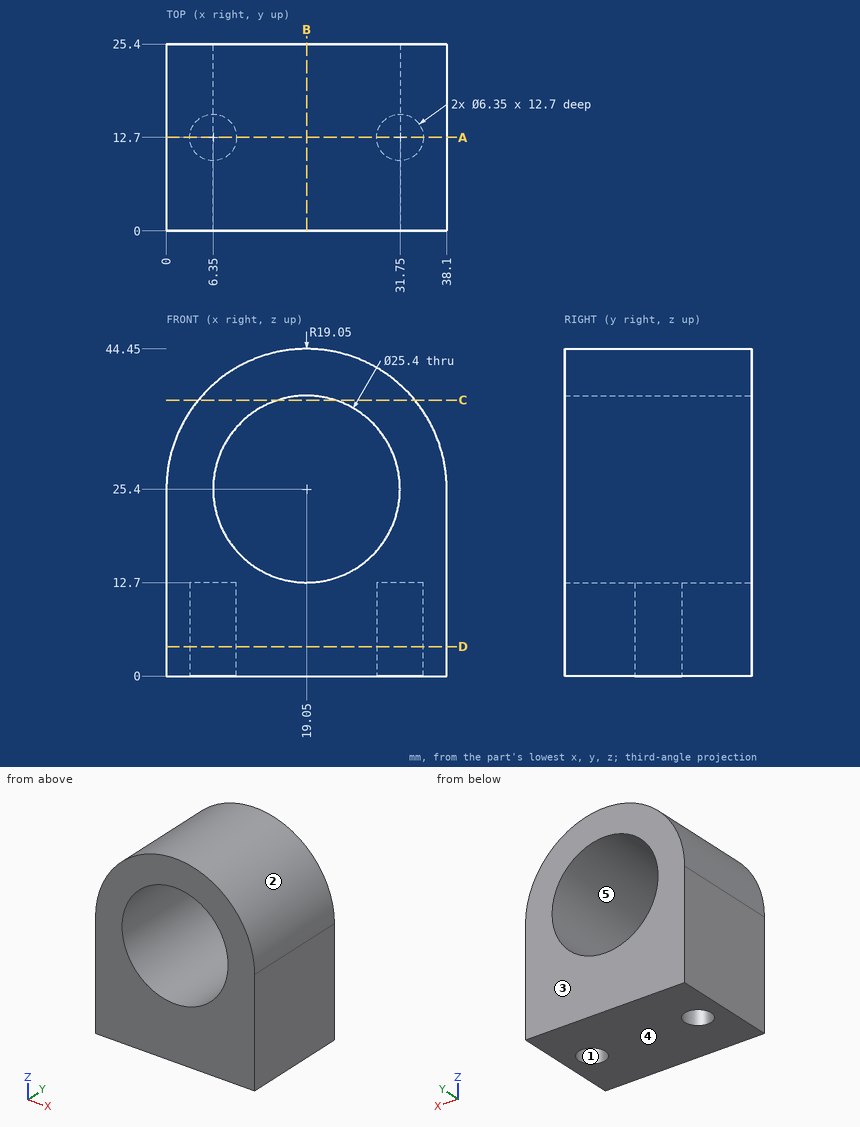
Geometry check sheet. Reference: drawing and pictorial views, mm from the part's lowest x, y, z. A direction names the side the tool comes from. Round coordinates to 2 decimals unless told otherwise and drop trailing zeros. Order: outer loops, then holes, each group sorted by start corner. A loop starts at its lowest first (then second) coordinate and runs counter-clockwise, first axis right, second up. Notation, with made-up numbers: M 22,-13.5 L 53,-13.5 A29 ccw 53,23.5 Z; hole C 42,49 d8. An arc over 180 degrees is marked long. One line per item, written item: value. Start each with the question number.
1. Gauge pin test, flat ends, axial feed: P1, Ø10, axis at x = 8, z = 20, coming from the -Y side; P2, Ø6, axis at x = 33.5, y = 11, coming from the +Z side (3 decimals); P3, Ø1, axis at x = 23, y = 18, coming from the +Z side (3 decimals); P4, Ø12, axis at x = 18, y = 14, coming from the +Z side. Record the tip position at first contact, or that the pin passes through.
2. Section check B-B on x = 19.05. Enter the section's corners in (y, z), and give its area (3 significant figures).
3. Section check C-C on z = 37.5. Enter the section's corners in (x, y), and give its area (3 significant figures).
4. Scan lines: line 1 along X through (y, z) = (12.7, 6.25) (3 decimals); line 2 along Y through (x, z) = (31.75, 7.5) (3 decimals); line 3 along Z through (x, y) = (19.05, 8.5). Record each from-to range of solid material in increasing order.
5. Section check A-A on y = 12.7. Enter the section's corners in (x, z) (3 decimals).
6. Section check D-D on z = 4. Enter the section's corners in (x, y) (3 decimals).
7. Access from +Z, -Z, +X, -X, +Y, -Y to the whole of each face (thin tool, end or side, straight path). Record for the marked faces 1 and 2.
8. Release check for a two-part mould opening along Z. For the marked faces 3, 4 and 5 record: released by +Z, released by -Z, zero draft, split by the parting line, or undercut.
Results found:
1. P1: y = 0
1. P2: z = 40.625
1. P3: z = 44.135
1. P4: z = 44.45
2. outline: M 0,0 L 25.4,0 L 25.4,12.7 L 0,12.7 Z; M 0,38.1 L 25.4,38.1 L 25.4,44.45 L 0,44.45 Z
2. area: 484 mm^2
3. outline: M 4.34,0 L 15.19,0 L 15.19,25.4 L 4.34,25.4 Z; M 22.91,0 L 33.76,0 L 33.76,25.4 L 22.91,25.4 Z
3. area: 551 mm^2
4. line 1: 0 to 3.175, 9.525 to 28.575, 34.925 to 38.1
4. line 2: 0 to 9.525, 15.875 to 25.4
4. line 3: 0 to 12.7, 38.1 to 44.45
5. outline: M 0,0 L 3.175,0 L 3.175,12.7 L 9.525,12.7 L 9.525,0 L 28.575,0 L 28.575,12.7 L 34.925,12.7 L 34.925,0 L 38.1,0 L 38.1,25.4 A19.05 ccw 0,25.4 Z; hole C 19.05,25.4 d25.4
6. outline: M 0,0 L 38.1,0 L 38.1,25.4 L 0,25.4 Z; hole C 6.35,12.7 d6.35; hole C 31.75,12.7 d6.35
7. face 1: -Z
7. face 2: +Z, +Y, -Y
8. face 3: zero draft
8. face 4: released by -Z
8. face 5: undercut
